Read the model definition and answer for the solid it produces. Units are mm, in the model's axes. Face numbers are marked on the shaded views. Round coordinates to 2 decimals unless told otherwise and drop trailing zeros. Order: outer loops, then holes, each group sorted by start corner. A loop starts at its lowest first (then second) coordinate and runs counter-clockwise, first axis right, second up. Notation, with made-up numbers: (64, 38.5) -> (97, 38.5) arc R17 cw to (97, 49.5) -> close; hole circle Ø1 at (-6, 4). An arc over 180 degrees is marked (long way). Use a Markdown table: item, result. Add a question column.
1. Consider L1, parallel to X at y = 8.9, z = 0; L2, parallel to X at y = 0.65, z = 0; L3, parallel to Y at x = -8, z = -11.5. Determine where each line is inside the solid, lowest interval first. Write a range as [from, to].
2. Section A-A, the plane z = -2.5 is taken. Give the vertices of the cut face in (x, y).
3. Section C-C, the plane x = -11 is taken. Give the vertices of the cut face in (y, z), then the cut area to 3 significant figures.
4. Section D-D, the plane y = 6 is taken. Give the vertices of the cut face in (x, z).
5. The mould has two halves that part along Z. Classify the marked faces 1, 2 and 3: +Z half, -Z half, draft (parallel to the pull), parting line (faces both ways), or undercut.
6. Section B-B, the plane x = 3.5 is taken. Give the vertices of the cut face in (y, z), then the cut area to 3 significant figures.
7. Given pin 1 (16.5 mm diameter, centred on x = -6, z = 2.5, fed in from -Y); pin 2 (4.5 mm diameter, centred on x = -0.11, z = 14.78, fed in from +Y); pin 3 (2.5 mm diameter, centred on x = -15, z = 0, fed in from +Y); pin 4 (12 mm diameter, centred on x = 7.5, z = 13, fed in from -Y), each flat-ended and moving along its own axis, determine where each tip first touches the part or whether it passes through.
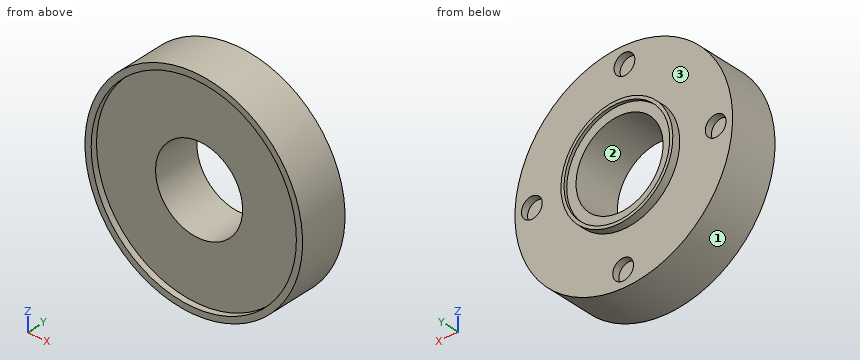
```python
from build123d import *

# Parameters (mm, degrees)
SKETCH1_R           = 17.5
BOSS_EXTRUDE1_DEPTH = 8
SKETCH5_R           = 16.5
CUT_EXTRUDE2_DEPTH  = 1
SKETCH11_R          = 1.67
CUT_EXTRUDE5_DEPTH  = 1.15
CIRPATTERN1_COUNT   = 4
SKETCH13_R          = 9
SKETCH13_R_2        = 8.5
BOSS_EXTRUDE3_DEPTH = 1.3
SKETCH12_R          = 8.6
BOSS_EXTRUDE2_DEPTH = 0.8
SKETCH14_R          = 7
CUT_EXTRUDE6_DEPTH  = 27.266708968


with BuildPart() as part:
    # Sketch1 → Boss-Extrude1 (new body)
    with BuildSketch(Plane(origin=(0, 0, 0), x_dir=(1, 0, 0), z_dir=(0, 1, 0))):
        with Locations(Location((0, 0, 0), (0, 0, 270))):
            Circle(SKETCH1_R)
    extrude(amount=BOSS_EXTRUDE1_DEPTH)

    # Sketch5 → Cut-Extrude2 (cut)
    with BuildSketch(Plane.XZ):
        with Locations(Location((0, 0, 0), (0, 0, 270))):
            Circle(SKETCH5_R)
    extrude(amount=-CUT_EXTRUDE2_DEPTH, mode=Mode.SUBTRACT)

    # Sketch11 → Cut-Extrude5 (cut)
    with BuildSketch(Plane(origin=(0, 8, 0), x_dir=(1, 0, 0), z_dir=(0, 1, 0))):
        with Locations(Location((0.106708516, 14.783412681, 0), (0, 0, 270))):
            Circle(SKETCH11_R)
    cut_extrude5 = extrude(amount=-CUT_EXTRUDE5_DEPTH, mode=Mode.SUBTRACT)

    # CirPattern1: Cut-Extrude5 ×4 about axis
    cirpattern1_axis = Axis((0, 0, 0), (0, 1, 0))
    for i in range(1, CIRPATTERN1_COUNT):
        add(cut_extrude5.rotate(cirpattern1_axis, i * 360 / CIRPATTERN1_COUNT), mode=Mode.SUBTRACT)

    # Sketch13 → Boss-Extrude3 (add)
    with BuildSketch(Plane(origin=(0, 8, 0), x_dir=(1, 0, 0), z_dir=(0, 1, 0))):
        with Locations(Location((0, 0, 0), (0, 0, 270))):
            Circle(SKETCH13_R)
        with Locations(Location((0, 0, 0), (0, 0, 270))):
            Circle(SKETCH13_R_2, mode=Mode.SUBTRACT)
    extrude(amount=BOSS_EXTRUDE3_DEPTH)

    # Sketch12 → Boss-Extrude2 (add)
    with BuildSketch(Plane(origin=(0, 8, 0), x_dir=(1, 0, 0), z_dir=(0, 1, 0))):
        Circle(SKETCH12_R)
    extrude(amount=BOSS_EXTRUDE2_DEPTH)

    # Sketch14 → Cut-Extrude6 (cut, through all)
    with BuildSketch(Plane(origin=(0, 8.8, 0), x_dir=(1, 0, 0), z_dir=(0, 1, 0))):
        with Locations(Location((0, 0, 0), (0, 0, 270))):
            Circle(SKETCH14_R)
    extrude(amount=-CUT_EXTRUDE6_DEPTH, mode=Mode.SUBTRACT)


solid = part.part
```
Verdict:
| question | item | result |
|---|---|---|
| 1 | L1 | x = [-9, -8.5], [8.5, 9] |
| 1 | L2 | x = [-17.5, -16.5], [16.5, 17.5] |
| 1 | L3 | y = [1, 8] |
| 2 | outline | (-17.32, 0) -> (-16.31, 0) -> (-16.31, 1) -> (-6.54, 1) -> (-6.54, 8.8) -> (-8.12, 8.8) -> (-8.12, 9.3) -> (-8.65, 9.3) -> (-8.65, 8) -> (-17.32, 8) -> close; (6.54, 1) -> (16.31, 1) -> (16.31, 0) -> (17.32, 0) -> (17.32, 8) -> (8.65, 8) -> (8.65, 9.3) -> (8.12, 9.3) -> (8.12, 8.8) -> (6.54, 8.8) -> close |
| 3 | outline | (0, -13.61) -> (8, -13.61) -> (8, 13.61) -> (0, 13.61) -> (0, 12.3) -> (1, 12.3) -> (1, -12.3) -> (0, -12.3) -> close |
| 3 | area | 193 mm2 |
| 4 | outline | circle Ø35 at (0, 0); hole circle Ø14 at (0, 0) |
| 5 | face 1 | parting line |
| 5 | face 2 | undercut |
| 5 | face 3 | draft |
| 6 | outline | (0, -17.15) -> (8, -17.15) -> (8, -8.29) -> (9.3, -8.29) -> (9.3, -7.75) -> (8.8, -7.75) -> (8.8, -6.06) -> (1, -6.06) -> (1, -16.12) -> (0, -16.12) -> close; (0, 16.12) -> (1, 16.12) -> (1, 6.06) -> (8.8, 6.06) -> (8.8, 7.75) -> (9.3, 7.75) -> (9.3, 8.29) -> (8, 8.29) -> (8, 17.15) -> (0, 17.15) -> close |
| 6 | area | 161 mm2 |
| 7 | pin 1 | stops at y = 1 |
| 7 | pin 2 | stops at y = 8 |
| 7 | pin 3 | stops at y = 6.85 |
| 7 | pin 4 | stops at y = 0 |
